Part model, mm, in its own coordinate system. Coordinates: 2 decimals unless noted, no trailing zeros. Write each loop counter-clockwise with the first axis right and the second up, starting at its lowest first coordinate (ties: lowest second). Pieces come first, ordered by that corner, then holes. Notation, with made-up numbers: M -4,73.25 L 51,73.25 A30 cw 51,102.25 Z; hole C -37,-36 d7. An arc over 180 degrees is marked long. Use a Markdown table: item, result. Add a question column.
Q1. Pin check, flat tips, straight feed: pin 1 Ø1 at (y, z) = (148.5, 11) entering from -X; pin 2 Ø1.9 at (x, y) = (197.74, 47.5) entering from -Z; pin 3 Ø4.5 at (y, z) = (9.5, 10) entering from -X. Stop position of each tip, or through.
Q2. Slice it at B-B on x = 178. Write the cut outline in (y, z).
Q3. Slice it at A-A on y = 189. Write the cut outline in (x, z), then the cut area to 3 significant figures.
Q4. Wall check: L1, parallel to X at y = -73.5, z = 9; L2, parallel to X at y = 106.23, z = 5.75; L3, parallel to Y at x = 302.5, z = 3. Give the ranges that are in metal, low to high. Write a range as from..to.
Q5. Slice it at C-C on z = 12.25. Count the separate pieces of the cut face and the enclosed holes in it, then the cut area to 3 significant figures.
from build123d import *

# Parameters (mm, degrees)
SKETCH_2_W          = 160.200177837
SKETCH_2_H          = 80
SKETCH_2_W_2        = 198.700177837
SKETCH_2_H_2        = 240
SKETCH_2_W_3        = 265
EXTRUDE_1_DEPTH     = 15
SKETCH_3_R          = 2.15
SKETCH_3_R_2        = 1.6
SKETCH_3_R_3        = 2.240696867
CUT_EXTRUDE_1_DEPTH = 15


with BuildPart() as part:
    # 草图2 → 凸台-拉伸1 (new body)
    with BuildSketch(Plane.XY):
        Polygon((-377.700177837, 310), (361.200177837, 310), (361.200177837, 40), (361.200177837, -40), (361.200177837, -310), (-377.700177837, -310), (-377.700177837, -175), (-322.700177837, -120), (-322.700177837, -40), (-322.700177837, 40), (-322.700177837, 120), (-377.700177837, 175), align=None)
        Polygon((-362.700177837, 295), (-147.5, 295), (-147.5, 55), (-307.700177837, 55), (-307.700177837, 126.213203436), (-362.700177837, 181.213203436), align=None, mode=Mode.SUBTRACT)
        with Locations((-227.600088919, 0)):
            Rectangle(SKETCH_2_W, SKETCH_2_H, mode=Mode.SUBTRACT)
        with Locations((246.850088919, 175)):
            Rectangle(SKETCH_2_W_2, SKETCH_2_H_2, mode=Mode.SUBTRACT)
        with Locations((0, 175)):
            Rectangle(SKETCH_2_W_3, SKETCH_2_H_2, mode=Mode.SUBTRACT)
        with Locations((246.850088919, -175)):
            Rectangle(SKETCH_2_W_2, SKETCH_2_H_2, mode=Mode.SUBTRACT)
        with Locations((0, -175)):
            Rectangle(SKETCH_2_W_3, SKETCH_2_H_2, mode=Mode.SUBTRACT)
        Polygon((-307.700177837, -126.213203436), (-307.700177837, -55), (-147.5, -55), (-147.5, -295), (-362.700177837, -295), (-362.700177837, -181.213203436), align=None, mode=Mode.SUBTRACT)
        Rectangle(SKETCH_2_W_3, SKETCH_2_H, mode=Mode.SUBTRACT)
        with Locations((246.850088919, 0)):
            Rectangle(SKETCH_2_W_2, SKETCH_2_H, mode=Mode.SUBTRACT)
    extrude(amount=EXTRUDE_1_DEPTH)

    # 草图3 → 切除-拉伸1 (cut)
    with BuildSketch(Plane.XY.offset(15)):
        with Locations((-140, 60)):
            Circle(SKETCH_3_R)
        with Locations((-315.200177837, 47.5)):
            Circle(SKETCH_3_R_2)
        with Locations((-256.466844504, 47.5)):
            Circle(SKETCH_3_R_2)
        with Locations((-197.736844504, 47.5)):
            Circle(SKETCH_3_R_2)
        with Locations((-140, 47.5)):
            Circle(SKETCH_3_R_2)
        with Locations((-140, 156.23)):
            Circle(SKETCH_3_R_2)
        with Locations((-140, 106.23)):
            Circle(SKETCH_3_R_2)
        with Locations((-81.27, 47.5)):
            Circle(SKETCH_3_R_2)
        with Locations((-22.54, 47.5)):
            Circle(SKETCH_3_R_2)
        with Locations((-140, 0)):
            Circle(SKETCH_3_R_3)
        with Locations((-302.700177837, 47.5)):
            Circle(SKETCH_3_R)
        with Locations(Location((-302.700177837, -47.5, 0), (0, 0, 180))):
            Circle(SKETCH_3_R)
        with Locations(Location((-22.54, -47.5, 0), (0, 0, 180))):
            Circle(SKETCH_3_R_2)
        with Locations(Location((-81.27, -47.5, 0), (0, 0, 180))):
            Circle(SKETCH_3_R_2)
        with Locations(Location((-140, -106.23, 0), (0, 0, 180))):
            Circle(SKETCH_3_R_2)
        with Locations(Location((-140, -156.23, 0), (0, 0, 180))):
            Circle(SKETCH_3_R_2)
        with Locations(Location((-140, -47.5, 0), (0, 0, 180))):
            Circle(SKETCH_3_R_2)
        with Locations(Location((-197.736844504, -47.5, 0), (0, 0, 180))):
            Circle(SKETCH_3_R_2)
        with Locations(Location((-256.466844504, -47.5, 0), (0, 0, 180))):
            Circle(SKETCH_3_R_2)
        with Locations(Location((-315.200177837, -47.5, 0), (0, 0, 180))):
            Circle(SKETCH_3_R_2)
        with Locations(Location((-140, -60, 0), (0, 0, 180))):
            Circle(SKETCH_3_R)
        with Locations((140, -60)):
            Circle(SKETCH_3_R)
        with Locations((256.466844504, -47.5)):
            Circle(SKETCH_3_R_2)
        with Locations((197.736844504, -47.5)):
            Circle(SKETCH_3_R_2)
        with Locations((140, -47.5)):
            Circle(SKETCH_3_R_2)
        with Locations((140, -156.23)):
            Circle(SKETCH_3_R_2)
        with Locations((140, -106.23)):
            Circle(SKETCH_3_R_2)
        with Locations((81.27, -47.5)):
            Circle(SKETCH_3_R_2)
        with Locations((22.54, -47.5)):
            Circle(SKETCH_3_R_2)
        with Locations((302.700177837, -47.5)):
            Circle(SKETCH_3_R)
        with Locations(Location((302.700177837, 47.5, 0), (0, 0, 180))):
            Circle(SKETCH_3_R)
        with Locations(Location((140, 0, 0), (0, 0, 180))):
            Circle(SKETCH_3_R_3)
        with Locations(Location((22.54, 47.5, 0), (0, 0, 180))):
            Circle(SKETCH_3_R_2)
        with Locations(Location((81.27, 47.5, 0), (0, 0, 180))):
            Circle(SKETCH_3_R_2)
        with Locations(Location((140, 106.23, 0), (0, 0, 180))):
            Circle(SKETCH_3_R_2)
        with Locations(Location((140, 156.23, 0), (0, 0, 180))):
            Circle(SKETCH_3_R_2)
        with Locations(Location((140, 47.5, 0), (0, 0, 180))):
            Circle(SKETCH_3_R_2)
        with Locations(Location((197.736844504, 47.5, 0), (0, 0, 180))):
            Circle(SKETCH_3_R_2)
        with Locations(Location((256.466844504, 47.5, 0), (0, 0, 180))):
            Circle(SKETCH_3_R_2)
        with Locations(Location((140, 60, 0), (0, 0, 180))):
            Circle(SKETCH_3_R)
    extrude(amount=-CUT_EXTRUDE_1_DEPTH, mode=Mode.SUBTRACT)


solid = part.part
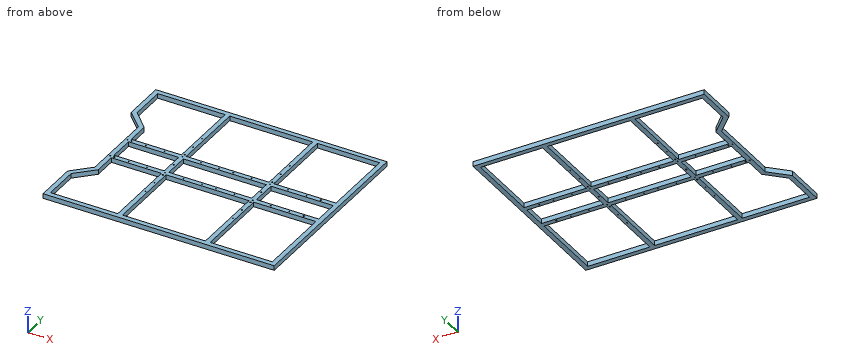
Recorded:
| question | item | result |
|---|---|---|
| 1 | pin 1 | x = -351.7 |
| 1 | pin 2 | through |
| 1 | pin 3 | x = -322.7 |
| 2 | outline | M -310,0 L -295,0 L -295,15 L -310,15 Z; M -55,0 L -40,0 L -40,15 L -55,15 Z; M 40,0 L 55,0 L 55,15 L 40,15 Z; M 295,0 L 310,0 L 310,15 L 295,15 Z |
| 3 | outline | M -377.7,0 L -362.7,0 L -362.7,15 L -377.7,15 Z; M -147.5,0 L -132.5,0 L -132.5,15 L -147.5,15 Z; M 132.5,0 L 147.5,0 L 147.5,15 L 132.5,15 Z; M 346.2,0 L 361.2,0 L 361.2,15 L 346.2,15 Z |
| 3 | area | 900 mm² |
| 4 | L1 | -322.7..-307.7, -147.5..-132.5, 132.5..147.5, 346.2..361.2 |
| 4 | L2 | -322.7..-307.7, -147.5..-141.6, -138.4..-132.5, 132.5..138.4, 141.6..147.5, 346.2..361.2 |
| 4 | L3 | -310..-295, -55..-49.64, -45.36..-40, 40..45.36, 49.64..55, 295..310 |
| 5 | separate pieces | 1 |
| 5 | enclosed holes | 49 |
| 5 | area | 76,600 mm² |
